Autodesk Inventor part; units mm, degrees
ref_plane "YZ Plane" through (0, 0, 0) normal (1, 0, 0) x (0, 1, 0)
ref_plane "XZ Plane" through (0, 0, 0) normal (0, 1, 0) x (-1, 0, 0)
ref_plane "XY Plane" through (0, 0, 0) normal (0, 0, 1) x (1, 0, 0)
sketch "Szkic1" plane through (0, 0, 0) normal (0, 0, 1) x (1, 0, 0)
  circle A0 centre (-27.3367, -1.5929) radius 18
  circle A1 centre (-27.3367, -1.5929) radius 38
  line L0 (-63.0867, 41.2281) -> (-70.1578, 34.1571)
  line L1 (8.4133, 41.2281) -> (15.4843, 34.1571)
  line L2 (-70.1578, -37.3429) -> (-63.0867, -44.414)
  line L3 (8.4133, -44.414) -> (15.4843, -37.3429)
  line L4 (-70.1578, 34.1571) -> (-57.5087, 21.508)
  line L5 (-70.1578, -37.3429) -> (-57.5087, -24.6938)
  line L6 (-63.0867, 41.2281) -> (-50.4376, 28.579)
  line L7 (-4.2358, 28.579) -> (8.4133, 41.2281)
  line L8 (2.8352, 21.508) -> (15.4843, 34.1571)
  line L9 (2.8352, -24.6938) -> (15.4843, -37.3429)
  line L10 (-4.2358, -31.7649) -> (8.4133, -44.414)
  line L11 (-63.0867, -44.414) -> (-50.4376, -31.7649)
  point P0 (0, 0)
  point P1 (-63.0867, 34.1571)
  point P2 (8.4133, 34.1571)
  point P3 (-63.0867, -37.3429)
  point P4 (8.4133, -37.3429)
  dimension "d5" = 76
  dimension "d0" = 71.5
  dimension "d1" = 71.5
  dimension "d2" = 35.75
  dimension "d3" = 35.75
  dimension "d4" = 36
  dimension "d14" = 5
  dimension "d15" = 5
  dimension "d16" = 5
  dimension "d17" = 5
extrude "Wyciągnięcie proste1" add sketch "Szkic1" along normal blind 2
hole "Otwór1" at (-63.0867, 34.1571, 0) at (8.4133, 34.1571, 0) at (-63.0867, -37.3429, 0) at (8.4133, -37.3429, 0) at (-27.3367, -1.5929, 0) direction (0, 0, 1) diameter 4 end through all
fillet "Zaokrąglenie1" radius 3 8 edges at (-63.0867, 41.2281, 1) (15.4843, 34.1571, 1) (8.4133, 41.2281, 1) (-70.1578, 34.1571, 1) (-63.0867, -44.414, 1) (-70.1578, -37.3429, 1) (15.4843, -37.3429, 1) (8.4133, -44.414, 1)
fillet "Zaokrąglenie1" radius 5 8 edges at (-57.5087, 21.508, 1) (-50.4376, 28.579, 1) (-57.5087, -24.6938, 1) (-50.4376, -31.7649, 1) (-4.2358, -31.7649, 1) (2.8352, -24.6938, 1) (-4.2358, 28.579, 1) (2.8352, 21.508, 1)
sketch "Szkic2" plane through (0, 0, 2) normal (0, 0, 1) x (1, 0, 0)
  circle A0 centre (8.4133, -37.3429) radius 2
  circle A1 centre (8.4133, 34.1571) radius 2
  circle A2 centre (-63.0867, 34.1571) radius 2
  circle A3 centre (-63.0867, -37.3429) radius 2
  circle A4 centre (-27.3367, -1.5929) radius 18
  arc A5 (6.2919, -42.2927) -> (10.5346, -42.2927) centre (8.4133, -40.1714) ccw
  line L0 (10.5346, -42.2927) -> (13.363, -39.4643)
  arc A6 (13.363, -39.4643) -> (13.363, -35.2216) centre (11.2417, -37.3429) ccw
  line L1 (13.363, -35.2216) -> (5.7707, -27.6293)
  arc A7 (5.0455, -21.4774) -> (5.7707, -27.6293) centre (9.3063, -24.0938) ccw
  arc A8 (5.0455, -21.4774) -> (5.0455, 18.2916) centre (-27.3367, -1.5929) ccw
  arc A9 (5.7707, 24.4435) -> (5.0455, 18.2916) centre (9.3063, 20.9079) ccw
  line L2 (5.7707, 24.4435) -> (13.363, 32.0357)
  arc A10 (13.363, 32.0357) -> (13.363, 36.2784) centre (11.2417, 34.1571) ccw
  line L3 (13.363, 36.2784) -> (10.5346, 39.1068)
  arc A11 (10.5346, 39.1068) -> (6.2919, 39.1068) centre (8.4133, 36.9855) ccw
  line L4 (6.2919, 39.1068) -> (-1.3003, 31.5145)
  arc A12 (-7.4522, 30.7893) -> (-1.3003, 31.5145) centre (-4.8359, 35.0501) ccw
  arc A13 (-7.4522, 30.7893) -> (-47.2212, 30.7893) centre (-27.3367, -1.5929) ccw
  arc A14 (-53.3731, 31.5145) -> (-47.2212, 30.7893) centre (-49.8376, 35.0501) ccw
  line L5 (-53.3731, 31.5145) -> (-60.9654, 39.1068)
  arc A15 (-60.9654, 39.1068) -> (-65.2081, 39.1068) centre (-63.0867, 36.9855) ccw
  line L6 (-65.2081, 39.1068) -> (-68.0365, 36.2784)
  arc A16 (-68.0365, 36.2784) -> (-68.0365, 32.0357) centre (-65.9152, 34.1571) ccw
  line L7 (-68.0365, 32.0357) -> (-60.4442, 24.4435)
  arc A17 (-59.7189, 18.2916) -> (-60.4442, 24.4435) centre (-63.9797, 20.9079) ccw
  arc A18 (-59.7189, 18.2916) -> (-59.7189, -21.4774) centre (-27.3367, -1.5929) ccw
  arc A19 (-60.4442, -27.6293) -> (-59.7189, -21.4774) centre (-63.9797, -24.0938) ccw
  line L8 (-60.4442, -27.6293) -> (-68.0365, -35.2216)
  arc A20 (-68.0365, -35.2216) -> (-68.0365, -39.4643) centre (-65.9152, -37.3429) ccw
  line L9 (-68.0365, -39.4643) -> (-65.2081, -42.2927)
  arc A21 (-65.2081, -42.2927) -> (-60.9654, -42.2927) centre (-63.0867, -40.1714) ccw
  line L10 (-60.9654, -42.2927) -> (-53.3731, -34.7004)
  arc A22 (-47.2212, -33.9751) -> (-53.3731, -34.7004) centre (-49.8376, -38.2359) ccw
  arc A23 (-47.2212, -33.9751) -> (-7.4522, -33.9751) centre (-27.3367, -1.5929) ccw
  arc A24 (-1.3003, -34.7004) -> (-7.4522, -33.9751) centre (-4.8359, -38.2359) ccw
  line L11 (-1.3003, -34.7004) -> (6.2919, -42.2927)
  line L12 (-27.3367, 32.9071) -> (-27.3367, 19.9071)
  arc A25 (-27.3367, 19.9071) -> (-32.3762, 32.1571) centre (-42.2339, 20.9402) ccw construction
  arc A26 (-25.8403, 19.8033) -> (-31.386, 33.2838) centre (-42.2339, 20.9402) ccw
  arc A27 (-28.8331, 20.0108) -> (-33.3664, 31.0303) centre (-42.2339, 20.9402) ccw
  arc A28 (-28.8331, 20.0108) -> (-25.8403, 19.8033) centre (-27.3367, 19.9071) ccw
  arc A29 (-31.386, 33.2838) -> (-33.3664, 31.0303) centre (-32.3762, 32.1571) ccw
  arc A30 (-41.2457, 15.0053) -> (-38.7025, 16.5965) centre (-39.9741, 15.8009) ccw
  arc A31 (-38.7025, 16.5965) -> (-51.1127, 24.2428) centre (-52.6334, 7.8804) ccw
  arc A32 (-39.9741, 15.8009) -> (-51.2515, 22.7493) centre (-52.6334, 7.8804) ccw construction
  arc A33 (-41.2457, 15.0053) -> (-51.3903, 21.2557) centre (-52.6334, 7.8804) ccw
  arc A34 (-51.1127, 24.2428) -> (-51.3903, 21.2557) centre (-51.2515, 22.7493) ccw
  arc A35 (-48.3456, 3.6598) -> (-47.2233, 6.442) centre (-47.7844, 5.0509) ccw
  arc A36 (-47.2233, 6.442) -> (-61.7578, 5.3335) centre (-53.3705, -8.7979) ccw
  arc A37 (-47.7844, 5.0509) -> (-60.9922, 4.0436) centre (-53.3705, -8.7979) ccw construction
  arc A38 (-48.3456, 3.6598) -> (-60.2266, 2.7536) centre (-53.3705, -8.7979) ccw
  arc A39 (-61.7578, 5.3335) -> (-60.2266, 2.7536) centre (-60.9922, 4.0436) ccw
  arc A40 (-47.4207, -9.692) -> (-48.1482, -6.7816) centre (-47.7844, -8.2368) ccw
  arc A41 (-48.1482, -6.7816) -> (-59.2552, -16.2215) centre (-44.1635, -22.7241) ccw
  arc A42 (-47.7844, -8.2368) -> (-57.8776, -16.8151) centre (-44.1635, -22.7241) ccw construction
  arc A43 (-47.4207, -9.692) -> (-56.5, -17.4086) centre (-44.1635, -22.7241) ccw
  arc A44 (-59.2552, -16.2215) -> (-56.5, -17.4086) centre (-57.8776, -16.8151) ccw
  arc A45 (-38.8245, -19.9503) -> (-41.1237, -18.0233) centre (-39.9741, -18.9868) ccw
  arc A46 (-41.1237, -18.0233) -> (-44.5608, -32.1889) centre (-28.5293, -28.5789) ccw
  arc A47 (-39.9741, -18.9868) -> (-43.0975, -31.8594) centre (-28.5293, -28.5789) ccw construction
  arc A48 (-38.8245, -19.9503) -> (-41.6341, -31.5299) centre (-28.5293, -28.5789) ccw
  arc A49 (-44.5608, -32.1889) -> (-41.6341, -31.5299) centre (-43.0975, -31.8594) ccw
  arc A50 (-25.8403, -23.1967) -> (-28.8331, -22.9892) centre (-27.3367, -23.0929) ccw
  arc A51 (-28.8331, -22.9892) -> (-23.2874, -36.4697) centre (-12.4395, -24.126) ccw
  arc A52 (-27.3367, -23.0929) -> (-22.2973, -35.3429) centre (-12.4395, -24.126) ccw construction
  arc A53 (-25.8403, -23.1967) -> (-21.3071, -34.2162) centre (-12.4395, -24.126) ccw
  arc A54 (-23.2874, -36.4697) -> (-21.3071, -34.2162) centre (-22.2973, -35.3429) ccw
  arc A55 (-13.4277, -18.1912) -> (-15.971, -19.7824) centre (-14.6993, -18.9868) ccw
  arc A56 (-15.971, -19.7824) -> (-3.5608, -27.4287) centre (-2.04, -11.0662) ccw
  arc A57 (-14.6993, -18.9868) -> (-3.422, -25.9351) centre (-2.04, -11.0662) ccw construction
  arc A58 (-13.4277, -18.1912) -> (-3.2831, -24.4416) centre (-2.04, -11.0662) ccw
  arc A59 (-3.5608, -27.4287) -> (-3.2831, -24.4416) centre (-3.422, -25.9351) ccw
  arc A60 (-6.3279, -6.8457) -> (-7.4501, -9.6279) centre (-6.889, -8.2368) ccw
  arc A61 (-7.4501, -9.6279) -> (7.0843, -8.5193) centre (-1.303, 5.612) ccw
  arc A62 (-6.889, -8.2368) -> (6.3187, -7.2294) centre (-1.303, 5.612) ccw construction
  arc A63 (-6.3279, -6.8457) -> (5.5531, -5.9395) centre (-1.303, 5.612) ccw
  arc A64 (7.0843, -8.5193) -> (5.5531, -5.9395) centre (6.3187, -7.2294) ccw
  arc A65 (-7.2527, 6.5062) -> (-6.5253, 3.5957) centre (-6.889, 5.0509) ccw
  arc A66 (-6.5253, 3.5957) -> (4.5817, 13.0357) centre (-10.51, 19.5382) ccw
  arc A67 (-6.889, 5.0509) -> (3.2041, 13.6292) centre (-10.51, 19.5382) ccw construction
  arc A68 (-7.2527, 6.5062) -> (1.8266, 14.2228) centre (-10.51, 19.5382) ccw
  arc A69 (4.5817, 13.0357) -> (1.8266, 14.2228) centre (3.2041, 13.6292) ccw
  arc A70 (-15.849, 16.7644) -> (-13.5497, 14.8374) centre (-14.6993, 15.8009) ccw
  arc A71 (-13.5497, 14.8374) -> (-10.1126, 29.003) centre (-26.1442, 25.3931) ccw
  arc A72 (-14.6993, 15.8009) -> (-11.576, 28.6735) centre (-26.1442, 25.3931) ccw construction
  arc A73 (-15.849, 16.7644) -> (-13.0394, 28.344) centre (-26.1442, 25.3931) ccw
  arc A74 (-10.1126, 29.003) -> (-13.0394, 28.344) centre (-11.576, 28.6735) ccw
  point P0 (0, 0)
  dimension "d29" = 13
  dimension "d30" = 21.5
  dimension "d31" = 3
  dimension "d34" = 360
extrude "Wyciągnięcie proste2" cut sketch "Szkic2" against normal through all contours A28 A27 A29 A26 | A33 A34 A31 A30 | A38 A39 A36 A35 | A43 A44 A41 A40 | A48 A49 A46 A45 | A53 A54 A51 A50 | A58 A59 A56 A55 | A63 A64 A61 A60 | A68 A69 A66 A65 | A73 A74 A71 A70
equation "\"d11\" = d10"
equation "\"d12\" = d10"
equation "\"d13\" = d12"
properties part number "3DP_ABS_Chamber_Fan_Cover"
Input: part model. Units: mm. Frame: model coordinates. A direction names the side the tool comes from. Coordinates: 2 decimals unless noted, no trailing zeros. Order: outer loops, then holes, each group sorted by start corner. A loop starts at its lowest first (then second) coordinate and runs counter-clockwise, first axis right, second up. Notation, with made-up numbers: M 61.5,55.25 L 68.5,55.25 A21 cw 68.5,70.25 Z; hole C 59,68 d2. An arc over 180 degrees is marked long. Answer in a Markdown table with one row per item.
(1) Contact query for a flat-ended pin moving along its axis: pin 1 Ø1 at (x, z) = (-22.5, 0.5) entering from +Y. Output: stop coordinate, or through.
Numbers:
| item | result |
|---|---|
| pin 1 | stops at y = 36.16 |
(2) Material intervals for line 1 (Y direction, x = -56, z = 0.55); line 2 (Y direction, x = -14.5, z = 1.5); line 3 (Y direction, x = -4, z = 0.45), sorted ascending. Write a range as [from, to].
Numbers:
| item | result |
|---|---|
| line 1 | y = [-37.33, -16.37], [-11.33, 4.38], [7.42, 34.14] |
| line 2 | y = [-37.36, -21.78], [-17.5, -14.21], [11.03, 14.31], [18.7, 34.17] |
| line 3 | y = [-33.31, -27.38], [-24.36, -10.6], [-7.55, 4.45], [7.79, 30.12] |
(3) Draft query along Y for faces 4 (the flat face through (11.93, 37.71, 0.99)), 5 (the cylindrical face through (-27.04, -39.59, 0.99)), 6 (the cylindrical face through (-45.32, -2.38, 0.99)). Return one class per face: pulls with the +Y half, pulls with the -Y half, needs draft (parallel to the pull), parting line crosses it, or undercut.
Numbers:
| item | result |
|---|---|
| face 4 | pulls with the +Y half |
| face 5 | pulls with the -Y half |
| face 6 | undercut |
(4) Section query A-A, the plane x = -43.5. Output: boundary loops of the cut face in (y, z), plus the area to 3 significant figures.
Numbers:
| item | result |
|---|---|
| outline | M -35.98,0 L -33.3,0 L -33.3,2 L -35.98,2 Z; M -21.8,0 L -9.51,0 L -9.51,2 L -21.8,2 Z; M 6.33,0 L 17.73,0 L 17.73,2 L 6.33,2 Z; M 21.54,0 L 32.8,0 L 32.8,2 L 21.54,2 Z |
| area | 75.3 mm^2 |
(5) Section query B-B, the plane z = 0.4. Give the number of separate pieces and of enclosed holes in the cut face, plus the area to 3 significant figures.
Numbers:
| item | result |
|---|---|
| separate pieces | 1 |
| enclosed holes | 15 |
| area | 3,700 mm^2 |
(6) Access query for faces 1 (the cylindrical face through (-4.3, 30.08, 1.01)), 2 (the cylindrical face through (-13.11, 22.14, 1.01)), 3 (the flat face through (9.51, -31.37, 0.99)). Directions: +Z, -Z, +X, -X, +Y, -Y. A direction counts if a zero-diameter tool reaches every point of the face in a straight line with its end or side. Return the directions, or none.
Numbers:
| item | result |
|---|---|
| face 1 | +Z, -Z, +Y |
| face 2 | +Z, -Z |
| face 3 | +Z, -Z, +X |
